```python
from build123d import *

# Parameters (mm, degrees)
SKETCH1_R           = 14.9225
BOSS_EXTRUDE1_DEPTH = 49.3268
BOSS_EXTRUDE2_DEPTH = 16.891
SKETCH3_R           = 17.399
BOSS_EXTRUDE3_DEPTH = 24.5872
SKETCH4_R           = 2.37871
BOSS_EXTRUDE4_DEPTH = 19.05
SKETCH5_R           = 6.35
BOSS_EXTRUDE5_DEPTH = 1.524
SKETCH6_R           = 1.190625
CUT_EXTRUDE1_DEPTH  = 19.05
CUT_EXTRUDE2_START  = -7.874
CUT_EXTRUDE2_DEPTH  = 7.874


with BuildPart() as part:
    # Sketch1 → Boss-Extrude1 (new body)
    with BuildSketch(Plane(origin=(0, 0, 0), x_dir=(0, 0, -1), z_dir=(1, 0, 0))):
        Circle(SKETCH1_R)
    extrude(amount=BOSS_EXTRUDE1_DEPTH)

    # Sketch2 → Boss-Extrude2 (add)
    with BuildSketch(Plane.ZY):
        with BuildLine():
            Line((-14.9225, 26.035), (14.9225, 26.035))
            Line((14.9225, 26.035), (14.9225, 0))
            ThreePointArc((14.9225, 0), (0, -14.9225), (-14.9225, 0))
            Line((-14.9225, 0), (-14.9225, 26.035))
        make_face()
    extrude(amount=-BOSS_EXTRUDE2_DEPTH)

    # Sketch3 → Boss-Extrude3 (add)
    with BuildSketch(Plane(origin=(49.3268, 0, 0), x_dir=(0, 0, -1), z_dir=(1, 0, 0))):
        Circle(SKETCH3_R)
    extrude(amount=BOSS_EXTRUDE3_DEPTH)

    # Sketch4 → Boss-Extrude4 (add)
    with BuildSketch(Plane(origin=(73.914, 0, 0), x_dir=(0, 0, -1), z_dir=(1, 0, 0))):
        with Locations(Location((0, 6.6548, 0), (0, 0, 180))):
            Circle(SKETCH4_R)
    extrude(amount=BOSS_EXTRUDE4_DEPTH)

    # Sketch5 → Boss-Extrude5 (add)
    with BuildSketch(Plane(origin=(73.914, 0, 0), x_dir=(0, 0, -1), z_dir=(1, 0, 0))):
        with Locations(Location((0, 6.6548, 0), (0, 0, 180))):
            Circle(SKETCH5_R)
    extrude(amount=BOSS_EXTRUDE5_DEPTH)

    # Sketch6 → Cut-Extrude1 (cut)
    with BuildSketch(Plane(origin=(73.914, 0, 0), x_dir=(0, 0, -1), z_dir=(1, 0, 0))):
        with Locations((3.490795989, -13.027827989)):
            Circle(SKETCH6_R)
        with Locations((-13.027827989, 3.490795989)):
            Circle(SKETCH6_R)
        with Locations((9.537032001, 9.537032001)):
            Circle(SKETCH6_R)
    extrude(amount=-CUT_EXTRUDE1_DEPTH, mode=Mode.SUBTRACT)

    # Sketch7 → Cut-Extrude2 (cut)
    with BuildSketch(Plane(origin=(92.964, 0, 0), x_dir=(0, 0, -1), z_dir=(1, 0, 0)).offset(CUT_EXTRUDE2_START)):
        with BuildLine():
            Line((-1.678707503, 8.34009), (1.678707503, 8.34009))
            ThreePointArc((1.678707503, 8.34009), (0, 9.03351), (-1.678707503, 8.34009))
        make_face()
    extrude(amount=CUT_EXTRUDE2_DEPTH, mode=Mode.SUBTRACT)


solid = part.part
```
The listing builds one solid part. Answer for the finished solid, in the listing's coordinates (mm). A direction names the side the tool comes from. Give positions to 0.01 mm unless a question says otherwise; leave off trailing zeros. Order: outer loops, then holes, each group sorted by start corner. A loop starts at its lowest first (then second) coordinate and runs counter-clockwise, first axis right, second up. Notation, with made-up numbers: (78.5, -34) -> (114.5, -34) arc R22 ccw to (114.5, -25) -> close; hole circle Ø4 at (45.25, -31.5). An arc over 180 degrees is marked (long way). Write each question's results on one line, items separated by ' | '.
Q1. The part is cut by section C-C, the plane y = 22.5. Give the vertices of the cut face in (x, z), and give its area (3 significant figures).
Checked values:
outline: (0, -14.92) -> (16.89, -14.92) -> (16.89, 14.92) -> (0, 14.92) -> close | area: 504 mm^2
Q2. The part is cut by section A-A, the plane z = 0. Give the vertices of the cut face in (x, y) (1 decimal), and give its area (3 significant figures).
Checked values:
outline: (0, -14.9) -> (49.3, -14.9) -> (49.3, -17.4) -> (73.9, -17.4) -> (73.9, 0.3) -> (75.4, 0.3) -> (75.4, 4.3) -> (93, 4.3) -> (93, 8.3) -> (85.1, 8.3) -> (85.1, 9) -> (75.4, 9) -> (75.4, 13) -> (73.9, 13) -> (73.9, 17.4) -> (49.3, 17.4) -> (49.3, 14.9) -> (16.9, 14.9) -> (16.9, 26) -> (0, 26) -> close | area: 2,610 mm^2
Q3. Straight lines are drawn through the part: probe 1 along Z at (x, y) = (15.5, 1.5); probe 2 along X at (y, z) = (6, 4.5); probe 3 along X at (y, z) = (12.5, 6). For each, find the intervals that lie inside material, in ascending order. Write a range as from..to.
Checked values:
probe 1: z = -14.92..14.92 | probe 2: x = 0..75.44 | probe 3: x = 0..73.91
Q4. The part is cut by section D-D, the plane x = 64. Give the vertices of the cut face in (y, z).
Checked values:
outline: circle Ø34.8 at (0, 0); hole circle Ø2.38 at (-13.03, -3.49); hole circle Ø2.38 at (3.49, 13.03); hole circle Ø2.38 at (9.54, -9.54)
Q5. Which of the six approach directions +Z, -Z, +X, -X, +Y, -Y give full straight-line access (tool end or side, diameter ignored) to faces 1 (the face through (49.327, 13, -8)), 2 (the face through (8, 13, -14.922)), 3 (the face through (64.522, 2.435, 12.478)), 4 (the face through (8, 13, 14.922))?
Checked values:
face 1: none | face 2: -Z, -X, +Y, -Y | face 3: +X | face 4: +Z, -X, +Y, -Y
Q6. The part is cut by section B-B, the plane x = 9. Give the vertices of the cut face in (y, z) (1 decimal), and give its area (3 significant figures).
Checked values:
outline: (0, -14.9) -> (26, -14.9) -> (26, 14.9) -> (0, 14.9) arc R14.9 ccw to start | area: 1,130 mm^2
Q7. Determine the mould class of faces 5 (the face through (64.522, -12.67, -4.626)), 6 (the face through (54.864, -13, -3)), 7 (the face through (29.799, -13.239, -6.886)) for opening direction X: pulls with the +X half, pulls with the -X half, needs draft (parallel to the pull), parting line crosses it, or undercut.
Checked values:
face 5: needs draft | face 6: pulls with the +X half | face 7: undercut
Q8. Each of these flat-tipped pins is pushed along its axis until it touches: P1, Ø0.7, axis at y = 9, z = -9.5, coming from the +X side; P2, Ø5, axis at x = 12, y = 14.5, coming from the -Z side; P3, Ø12, axis at x = 27, z = -9.5, coming from the +Y side; P4, Ø17.5, axis at y = -5, z = 7.5, coming from the -X side. Where does it stop, or does it pass through?
Checked values:
P1: stops at x = 54.86 | P2: stops at z = -14.92 | P3: stops at y = 14.51 | P4: stops at x = 0
